Input: part model. Units: mm. Frame: model coordinates. Give positions to 0.01 mm unless a question says otherwise; leave off trailing zeros. Loops run counter-clockwise (first coordinate to the right, second up) from the corner with the lowest first, then second, coordinate; pieces in that order, holes last. Notation, with made-up numbers: M 32,64 L 48,64 A7 cw 48,71 Z; hole C 16.5,-23.5 d5. An arc over 180 degrees is marked long. Use CSV: the item, a comma, the result in double quotes. Start each with the question number.
Q1. Section A-A, the plane z = -40.5. Output: boundary loops of the cut face in (x, y).
Q2. Material intervals for line 1 along Z through (x, y) = (0, -0.4); line 2 along X through (y, z) = (2.5, 83.5); line 3 along X through (y, z) = (1.25, -54.5), sorted ascending.
Q3. Pin query (flat end, axial travel): pin 1 (5 mm diameter, centred on x = 0, z = -140, fed in from +Y). Return the tip coordinate at first contact, or that it passes through.
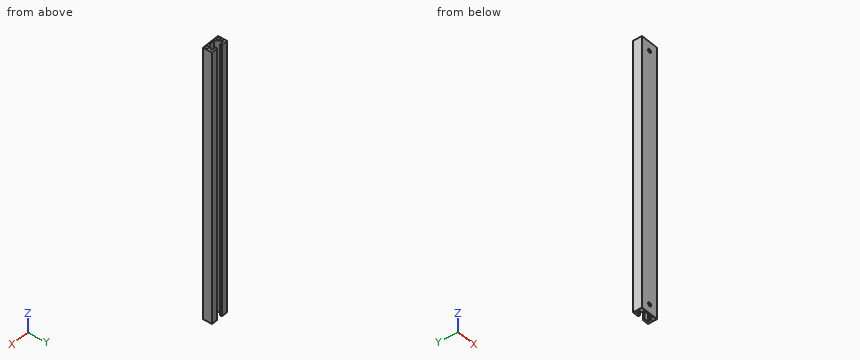
from build123d import *

# Parameters (mm, degrees)
BOSS_EXTRUDE1_DEPTH = 150
SKETCH2_R           = 1.9
CUT_EXTRUDE1_DEPTH  = 301.290281321
SKETCH3_R           = 2
CUT_EXTRUDE2_DEPTH  = 10


with BuildPart() as part:
    # Sketch1 → Boss-Extrude1 (new, symmetric)
    with BuildSketch(Plane.XY):
        Polygon((0, 0), (0, -1.382978723), (10, -1.382978723), (10, 8.617021277), (3.448211747, 8.617021277), (3, 8.117021277), (3, 6.617021277), (7.587018089, 6.617021277), (7.587018089, 5.117021277), (3, 0), align=None)
    boss_extrude1 = extrude(amount=BOSS_EXTRUDE1_DEPTH, both=True)

    # Mirror1: Boss-Extrude1 across plane
    add(boss_extrude1.mirror(Plane(origin=(0, 0, 0), x_dir=(0, 0, 1), z_dir=(1, 0, 0))))

    # Sketch2 → Cut-Extrude1 (cut, through all)
    with BuildSketch(Plane.XY.offset(150)):
        with Locations((7.646716257, 0.97030502)):
            Circle(SKETCH2_R)
    cut_extrude1 = extrude(amount=-CUT_EXTRUDE1_DEPTH, mode=Mode.SUBTRACT)

    # Mirror2: Cut-Extrude1 across plane
    add(cut_extrude1.mirror(Plane(origin=(0, 0, 0), x_dir=(0, 0, 1), z_dir=(1, 0, 0))), mode=Mode.SUBTRACT)

    # Sketch3 → Cut-Extrude2 (cut)
    with BuildSketch(Plane(origin=(0, 0, 0), x_dir=(1, 0, 0), z_dir=(0, 1, 0))):
        with Locations(Location((0, -140, 0), (0, 0, 180))):
            Circle(SKETCH3_R)
    cut_extrude2 = extrude(amount=-CUT_EXTRUDE2_DEPTH, mode=Mode.SUBTRACT)

    # Mirror3: Cut-Extrude2 across plane
    add(cut_extrude2.mirror(Plane.XY), mode=Mode.SUBTRACT)


solid = part.part
A:
1,outline,"M -10,-1.38 L 10,-1.38 L 10,8.62 L 3.45,8.62 L 3,8.12 L 3,6.62 L 7.59,6.62 L 7.59,5.12 L 3,0 L -3,0 L -7.59,5.12 L -7.59,6.62 L -3,6.62 L -3,8.12 L -3.45,8.62 L -10,8.62 Z; hole C -7.65,0.97 d3.8; hole C 7.65,0.97 d3.8"
2,line 1,"-150 to -142, -138 to 138, 142 to 150"
2,line 2,"-10 to -8.77, -6.52 to -5.24, 5.24 to 6.52, 8.77 to 10"
2,line 3,"-10 to -9.53, -5.77 to -4.12, 4.12 to 5.77, 9.53 to 10"
3,pin 1,"y = 0"
